Autodesk Inventor part; units mm, degrees
ref_plane "YZ Plane" through (0, 0, 0) normal (1, 0, 0) x (0, 1, 0)
ref_plane "XZ Plane" through (0, 0, 0) normal (0, 1, 0) x (-1, 0, 0)
ref_plane "XY Plane" through (0, 0, 0) normal (0, 0, 1) x (1, 0, 0)
sketch "スケッチ1" plane through (0, 0, 0) normal (0, 0, 1) x (1, 0, 0)
  circle A0 centre (0, 0) radius 5 construction
  line L0 (-60, 11) -> (-50.7483, 11)
  line L1 (60, 11) -> (60, 5)
  line L2 (60, 5) -> (34, 5)
  line L3 (34, 5) -> (34, -5)
  line L4 (34, -5) -> (60, -5)
  line L5 (60, -5) -> (60, -11)
  line L6 (60, -11) -> (50.7483, -11)
  line L7 (-60, -11) -> (-60, -5)
  line L8 (-60, -5) -> (-34, -5)
  line L9 (-34, -5) -> (-34, 5)
  line L10 (-34, 5) -> (-60, 5)
  line L11 (-60, 5) -> (-60, 11)
  arc A1 (-49.2517, 11) -> (-50.7483, 11) centre (-50, 12.3) ccw construction
  arc A2 (50.7483, 11) -> (49.2517, 11) centre (50, 12.3) ccw construction
  arc A3 (-50.7483, -11) -> (-49.2517, -11) centre (-50, -12.3) ccw construction
  arc A4 (49.2517, -11) -> (50.7483, -11) centre (50, -12.3) ccw construction
  arc A5 (-50.7483, 11) -> (-49.2517, 11) centre (-50, 12.3) ccw
  line L12 (-49.2517, 11) -> (49.2517, 11)
  line L13 (-50.7483, 11) -> (-49.2517, 11) construction
  line L14 (-49.2517, -11) -> (-50.7483, -11) construction
  line L15 (-50.7483, -11) -> (-60, -11)
  arc A6 (-49.2517, -11) -> (-50.7483, -11) centre (-50, -12.3) ccw
  arc A7 (49.2517, 11) -> (50.7483, 11) centre (50, 12.3) ccw
  line L16 (50.7483, 11) -> (60, 11)
  line L17 (49.2517, 11) -> (50.7483, 11) construction
  arc A8 (50.7483, -11) -> (49.2517, -11) centre (50, -12.3) ccw
  line L18 (50.7483, -11) -> (49.2517, -11) construction
  line L19 (49.2517, -11) -> (-49.2517, -11)
  dimension "d0" = 10
  dimension "d1" = 10
  dimension "d2" = 10
  dimension "d3" = 5
  dimension "d4" = 5
  dimension "d5" = 6
  dimension "d6" = 6
  dimension "d7" = 3
  dimension "d8" = 3
  dimension "d9" = 3
  dimension "d10" = 3
  dimension "d11" = 1.3
  dimension "d12" = 1.3
  dimension "d13" = 1.3
  dimension "d14" = 1.3
  dimension "d15" = 100
  dimension "d17" = 50
  dimension "d19" = 16
  dimension "d20" = 10
  dimension "d21" = 10
  dimension "d22" = 16
extrude "押し出し1" add sketch "スケッチ1" along normal blind 10
sketch "スケッチ2" plane through (-49.2517, 11, 0) normal (0, 1, 0) x (1, 0, 0)
  circle A0 centre (-0.7483, -5) radius 3.05
  circle A1 centre (99.2517, -5) radius 3.05
  line L0 (-10.7483, 0) -> (-10.7483, -10)
  point P0 (49.2517, 0)
  point P1 (-10.7483, -5)
  dimension "d26" = 6.1
  dimension "d27" = 6.1
  dimension "d28" = 50
  dimension "d29" = 50
extrude "押し出し2" cut sketch "スケッチ2" against normal through all
fillet "フィレット1" radius 3 12 edges at (-34, 5, 5) (-34, -5, 5) (34, 5, 5) (34, -5, 5) (-60, 11, 5) (-60, 5, 5) (-60, -5, 5) (-60, -11, 5) (60, 11, 5) (60, 5, 5) (60, -5, 5) (60, -11, 5)
sketch "スケッチ4" plane through (0, 0, 10) normal (0, 0, 1) x (1, 0, 0)
  point P0 (0, 0)
hole "穴1" at (0, 0, 10) direction (0, 0, -1) diameter 8.647 end through all
properties part number "ハンド_ピストン先" material "ポリカーボネート、スモーク"
Check sheet for the modelled part. Datum: model origin and axes. Units: mm. A direction names the side the tool comes from. Coordinates: 2 decimals unless noted, no trailing zeros. Order: outer loops, then holes, each group sorted by start corner. A loop starts at its lowest first (then second) coordinate and runs counter-clockwise, first axis right, second up. Notation, with made-up numbers: M -2,28 L 24,28 A25 ccw 24,58 Z; hole C 21.25,84.5 d9. An arc over 180 degrees is marked long. Write each question's results on one line, items separated by ' | '. Start each with the question number.
1. Cross-section at C-C on z = 5. State how many separate pieces and enclosed holes the cut face has, and give its area (3 significant figures).
2. Cross-section at A-A on y = 0. Record the cut outline in (x, z), and give its area (3 significant figures).
3. Cross-section at B-B on x = 0. Record the cut outline in (y, z), and give its area (3 significant figures).
4. Mould release check, pull along Y, two halves, no side actions. Record for faces 1 (the face through (45, 5, 5)), 2 (the face through (47.58, -7.958, 6.856)), 3 (the face through (55, -11, 5)): +Y half, -Y half, draft (parallel to the pull), parting line (faces both ways), or undercut.
5. Go/stop test with flat-tipped pins: P1, Ø6, axis at y = 3, z = 5.5, coming from the +X side; P2, Ø4.5, axis at y = -1, z = 5.5, coming from the -X side; P3, Ø2, axis at y = -4.5, z = 7.5, coming from the -X side. Record where each tip stops, or that it passes through.
6. Material ranges on probe 1 along Y at (x, z) = (-46.5, 1.25); probe 2 along X at (y, z) = (0, 3.5); probe 3 along X at (y, z) = (-6.5, 2.25), recorded low to high.
7. Access from +Z, -Z, +X, -X, +Y, -Y to the whole of each face (thin tool, end or side, straight path). Record for faces 4 (the face through (55, 11, 5)), 5 (the face through (59.1, 5.86, 5.07)), 6 (the face through (-45, -5, 5)).
Checks:
1) separate pieces: 5 | enclosed holes: 1 | area: 1,910 mm²
2) outline: M -34,0 L -4.32,0 L -4.32,10 L -34,10 Z; M 4.32,0 L 34,0 L 34,10 L 4.32,10 Z | area: 594 mm²
3) outline: M -11,0 L -4.32,0 L -4.32,10 L -11,10 Z; M 4.32,0 L 11,0 L 11,10 L 4.32,10 Z | area: 134 mm²
4) face 1: undercut | face 2: draft | face 3: -Y half
5) P1: stops at x = 59.24 | P2: stops at x = -34.27 | P3: stops at x = -58.66
6) probe 1: y = -11 to -5, 5 to 11 | probe 2: x = -34 to -4.32, 4.32 to 34 | probe 3: x = -59.6 to -51.32, -48.68 to 48.68, 51.32 to 59.6
7) face 4: +Z, -Z, +X, -X, +Y | face 5: +Z, -Z, +X | face 6: +Z, -Z, -X
